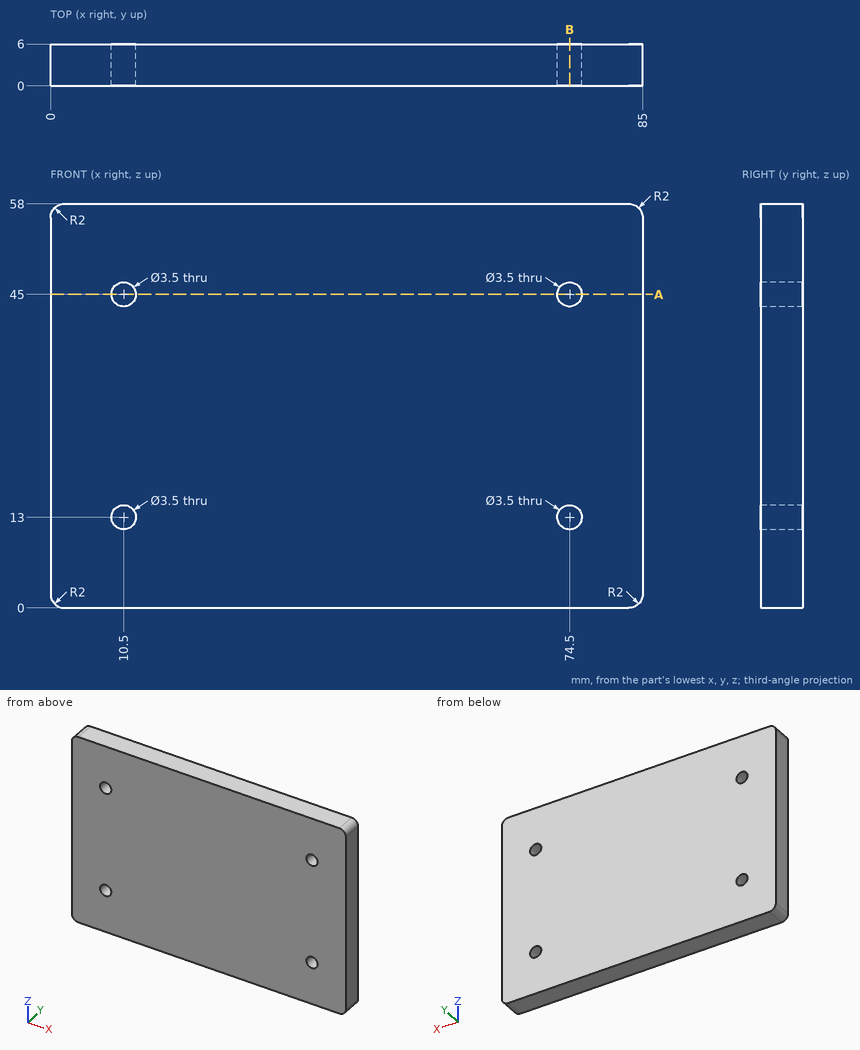
Answer from the drawing. Dimensions are ordinates in mm from the lowest x, y and z of the part. Give positions to 0.01 mm unless a question says otherwise; leave off trailing zeros. Loops run counter-clockwise (first coordinate to the right, second up) from the corner with the lowest first, then second, coordinate; pieces in that order, holes last.
Item 1: The part is cut by section A-A (z = 45). Write down the section's boundary in (x, y), and give its area (3 significant figures).
Item 2: The part is cut by section B-B (x = 74.5). Write down the section's boundary in (y, z).
Item 3: This flat-tipped pin is pushed along its axis until it touches: pin 1 Ø2 at (x, z) = (10.5, 13) entering from -Y. Where does it stop, or does it pass through?
Item 4: Find the intervals of material crossed by line 1 along X through (y, z) = (1.45, 45); line 2 along Z through (x, y) = (10.5, 2.85), in increasing order.
Taken from the geometry:
1. outline: (0, 0) - (8.75, 0) - (8.75, 6) - (0, 6) - close; (12.25, 0) - (72.75, 0) - (72.75, 6) - (12.25, 6) - close; (76.25, 0) - (85, 0) - (85, 6) - (76.25, 6) - close
1. area: 468 mm2
2. outline: (0, 0) - (6, 0) - (6, 11.25) - (0, 11.25) - close; (0, 14.75) - (6, 14.75) - (6, 43.25) - (0, 43.25) - close; (0, 46.75) - (6, 46.75) - (6, 58) - (0, 58) - close
3. pin 1: passes through
4. line 1: x = 0 to 8.75, 12.25 to 72.75, 76.25 to 85
4. line 2: z = 0 to 11.25, 14.75 to 43.25, 46.75 to 58
